The model under review builds one solid part; all positions refer to its coordinate system, in mm. A direction names the side the tool comes from. Give positions to 0.01 mm unless a question says otherwise; leave off trailing zeros. Order: outer loops, then holes, each group sorted by start corner. A loop starts at its lowest first (then second) coordinate and runs counter-clockwise, first axis right, second up. Notation, with made-up numbers: (27.25, 44.5) - (67.25, 44.5) arc R22 cw to (67.25, 74.5) - close; hole circle Ø3 at (82, 9). An arc over 180 degrees is marked (long way). Put each result on its own line as item: value.
```python
from build123d import *

# Parameters (mm, degrees)
SKETCH1_W             = 230
SKETCH1_H             = 66
BOSS_EXTRUDE1_DEPTH   = 4.5
SKETCH11_W            = 150
SKETCH11_H            = 66
BOSS_EXTRUDE2_DEPTH   = 4.5
F_5_0MM_DOWEL_HOLE1_D = 5
FILLET1_R             = 2


with BuildPart() as part:
    # Sketch1 → Boss-Extrude1 (new body)
    with BuildSketch(Plane(origin=(0, 0, 0), x_dir=(1, 0, 0), z_dir=(0, 1, 0))):
        with Locations((82.410138249, 12.451612903)):
            Rectangle(SKETCH1_W, SKETCH1_H)
    extrude(amount=BOSS_EXTRUDE1_DEPTH)

    # Sketch11 → Boss-Extrude2 (add)
    with BuildSketch(Plane(origin=(0, 4.5, 0), x_dir=(1, 0, 0), z_dir=(0, 1, 0))):
        with Locations((122.410138249, 12.451612903)):
            Rectangle(SKETCH11_W, SKETCH11_H)
    extrude(amount=BOSS_EXTRUDE2_DEPTH)

    # Ø5.0mm Dowel Hole1 (through all)
    with Locations(Plane(origin=(0, 0, 0), x_dir=(-1, 0, 0), z_dir=(0, -1, 0))):
        with Locations((5.923195084, 12.451612903), (-20.743471582, 12.451612903)):
            Hole(F_5_0MM_DOWEL_HOLE1_D / 2)

    # Fillet1
    fillet1_edges = [part.edges().sort_by_distance(p)[0] for p in [
        (122.410138249, 9, -45.451612903),
        (122.410138249, 9, 20.548387097),
        (197.410138249, 9, -12.451612903),
        (82.410138249, 0, -45.451612903),
        (197.410138249, 0, -12.451612903),
        (82.410138249, 0, 20.548387097),
    ]]
    fillet(fillet1_edges, radius=FILLET1_R)


solid = part.part
```
(1) The part is to be moulded in two halves that separate along X. For faces 1 (the flat face through (197.41, 4, -12)), 2 (the cylindrical face through (21.897, 2.281, -10.234)), 3 (the flat face through (-32.59, 2, -12)), 4 (the flat face through (7, 4.5, -13)), say which applies: pulls with the +X half, pulls with the -X half, needs draft (parallel to the pull), parting line crosses it, or undercut.
The answers:
face 1: pulls with the +X half
face 2: undercut
face 3: pulls with the -X half
face 4: needs draft
(2) Take a section at B-B, the plane x = 43. Write out the cut boundary in (y, z), then the cut area to 3 significant figures.
The answers:
outline: (0, -43.45) arc R2 ccw to (2, -45.45) - (4.5, -45.45) - (4.5, 20.55) - (2, 20.55) arc R2 ccw to (0, 18.55) - close
area: 295 mm^2
(3) Clearance check with flat-ended pins moving along their axes: pin 1 Ø8 at (x, z) = (-5.92, -12.45) entering from +Y; pin 2 Ø6.5 at (x, z) = (20.74, -12.45) entering from -Y; pin 3 Ø1.3 at (y, z) = (6, -5) entering from -X; pin 4 Ø1 at (x, y) = (46, 7) entering from -Z. State where each tip first meets the part, or that it passes through.
The answers:
pin 1: y = 4.5
pin 2: y = 0
pin 3: x = 47.41
pin 4: through
(4) Wall thickness on L1, parallel to X at y = 4.75, z = -22.5; L2, parallel to Y at x = 34.5, z = -36.5; L3, parallel to X at y = 2.5, z = -14.5: over which ranges is each line inside the solid? List them lowest first.
The answers:
L1: 47.41 to 197.41
L2: 0 to 4.5
L3: -32.59 to -7.36, -4.49 to 19.31, 22.18 to 197.41
(5) For faces 5 (the flat face through (106, 4, -45.452)), 6 (the flat face through (47.41, 7, -12)), list the 3-axis set-ups (+Z, -Z, +X, -X, +Y, -Y) from which the entire face can be reached by the end or side of a thin tool; tool diameter is ignored.
The answers:
face 5: -Z, +X, -X, +Y, -Y
face 6: +Z, -Z, -X, +Y
(6) Take a section at A-A, the plane z = -20. Write out the cut boundary in (x, y), then the cut area to 3 significant figures.
The answers:
outline: (-32.59, 0) - (195.41, 0) arc R2 ccw to (197.41, 2) - (197.41, 7) arc R2 ccw to (195.41, 9) - (47.41, 9) - (47.41, 4.5) - (-32.59, 4.5) - close
area: 1,710 mm^2
